Read the model definition and answer for the solid it produces. Units are mm, in the model's axes. A direction names the side the tool comes from. Coordinates: 2 decimals unless noted, no trailing zeros. Write each loop counter-clockwise with the first axis right and the second up, starting at its lowest first coordinate (ties: lowest second). Pieces come first, ordered by that corner, then holes.
(1) The part is cut by section A-A, the plane x = -9.5. Determine the outline of the cut face in (y, z).
(2) Which of the six approach directions +Z, -Z, +X, -X, +Y, -Y give full straight-line access (tool end or side, diameter ignored) to faces 1 (the flat face through (1, -8, -42)), 2 (the flat face through (50, -8.2, -25))?
(3) The part is cut by section C-C, the plane z = -11.5. Determine the outline of the cut face in (x, y).
(4) Straight lines are drawn through the part: line 1 along Y through (x, z) = (-23, -30); line 2 along Z through (x, y) = (-2, 6); line 3 along Z through (x, y) = (23, 7.75). For each, find the intervals that lie inside material, in ascending order.
(5) Given pin 1 (5 mm diameter, centred on x = -7, y = 0.5, fed in from -Z); pin 2 (12 mm diameter, centred on y = 2.5, z = -62.5, fed in from -X); pin 3 (2 mm diameter, centred on x = -6.5, y = 9, fed in from -Z), each flat-ended and moving along its own axis, determine where each tip first touches the part or whether it passes through.
(6) Determine the mould class of faces 3 (the cylindrical face through (0.7, -8.797, 8.859)), 4 (the flat face through (1, 0, 8)), 5 (the flat face through (1, 0, 10)), 6 (the flat face through (1, 8, -1)) for opening direction Y: pulls with the +Y half, pulls with the -Y half, needs draft (parallel to the pull), parting line crosses it, or undercut.
(7) The part is cut by section B-B, the plane y = 3.25. Determine the outline of the cut face in (x, z).
```python
from build123d import *

# Parameters (mm, degrees)
F1_DEPTH = 50


with BuildPart() as f1:
    # F0 (on Right) → F1 (new body, symmetric)
    with BuildSketch(Plane.YZ):
        with BuildLine():
            Line((6, 10), (-6, 10))
            ThreePointArc((-6, 10), (-8.828427, 8.828427), (-10, 6))
            Line((-10, 6), (-10, -10))
            Line((-10, -10), (-10, -90))
            Line((-10, -90), (-8, -90))
            Line((-8, -90), (-8, -10))
            Line((-8, -10), (-8, 8))
            Line((-8, 8), (8, 8))
            Line((8, 8), (8, -10))
            Line((8, -10), (10, -10))
            Line((10, -10), (10, 6))
            ThreePointArc((10, 6), (8.828427, 8.828427), (6, 10))
        make_face()
    extrude(amount=F1_DEPTH, both=True)


solid = f1.part
```
Computed:
1. outline: (-10, -90) - (-8, -90) - (-8, 8) - (8, 8) - (8, -10) - (10, -10) - (10, 6) arc R4 ccw to (6, 10) - (-6, 10) arc R4 ccw to (-10, 6) - close
2. face 1: -Z, +X, -X
2. face 2: +Z, -Z, +X, +Y, -Y
3. outline: (-50, -10) - (50, -10) - (50, -8) - (-50, -8) - close
4. line 1: y = -10 to -8
4. line 2: z = 8 to 10
4. line 3: z = 8 to 9.6
5. pin 1: stops at z = 8
5. pin 2: passes through
5. pin 3: stops at z = -10
6. face 3: pulls with the -Y half
6. face 4: undercut
6. face 5: needs draft
6. face 6: undercut
7. outline: (-50, 8) - (50, 8) - (50, 10) - (-50, 10) - close
